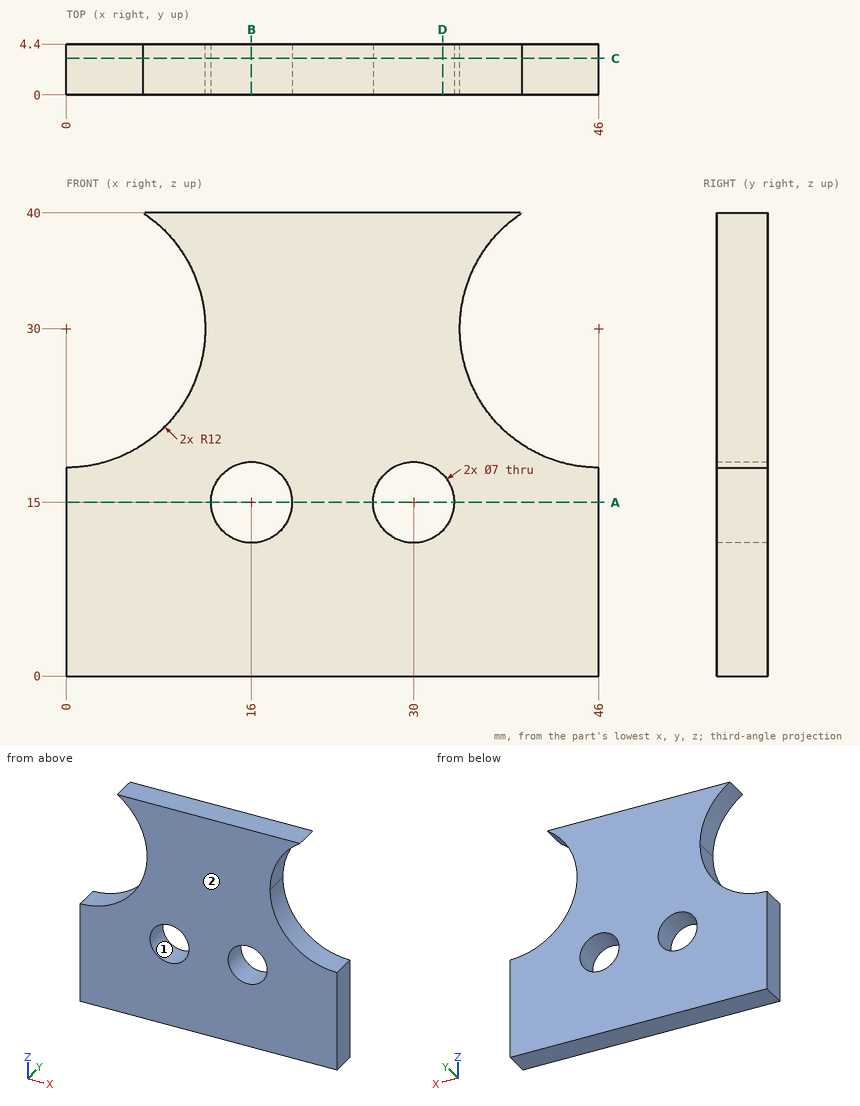
Print and shaded views of the part. All mm, measured from the part's lowest x, y and z. Round coordinates to 2 decimals unless told otherwise and drop trailing zeros. Write each loop counter-clockwise with the first axis right and the second up, starting at its lowest first coordinate (ties: lowest second). Pieces come first, ordered by that corner, then holes.
Item 1: Two-plate mould, pull along X, no slides. Class the marked faces 1 and 2: +X half, -X half, draft (parallel to the pull), parting line (faces both ways), or undercut.
Results:
face 1: undercut
face 2: draft
Item 2: Cut at B-B, the plane x = 16. Give the cut face in (y, z).
Results:
outline: (0, 0) - (4.4, 0) - (4.4, 11.5) - (0, 11.5) - close; (0, 18.5) - (4.4, 18.5) - (4.4, 40) - (0, 40) - close
Item 3: Probe L1, parallel to X at y = 3.5, z = 15; L2, parallel to Z at x = 37, y = 1.55; L3, parallel to Z at x = 8.5, y = 1.2. List the from-to ranges inside material, lowest first.
Results:
L1: x = 0 to 12.5, 19.5 to 26.5, 33.5 to 46
L2: z = 0 to 22.06, 37.94 to 40
L3: z = 0 to 21.53, 38.47 to 40
Item 4: Cut at A-A, the plane z = 15. Give the cut face in (x, y), plus the area to 3 significant figures.
Results:
outline: (0, 0) - (12.5, 0) - (12.5, 4.4) - (0, 4.4) - close; (19.5, 0) - (26.5, 0) - (26.5, 4.4) - (19.5, 4.4) - close; (33.5, 0) - (46, 0) - (46, 4.4) - (33.5, 4.4) - close
area: 141 mm2
Item 5: Cut at D-D, the plane x = 32.5. Give the cut face in (y, z), plus the area to 3 significant figures.
Results:
outline: (0, 0) - (4.4, 0) - (4.4, 12.55) - (0, 12.55) - close; (0, 17.45) - (4.4, 17.45) - (4.4, 40) - (0, 40) - close
area: 154 mm2
Item 6: Cut at C-C, the plane y = 3.15. Give the cut face in (x, z), plus the area to 3 significant figures.
Results:
outline: (0, 0) - (46, 0) - (46, 18) arc R12 cw to (39.37, 40) - (6.63, 40) arc R12 cw to (0, 18) - close; hole circle Ø7 at (16, 15); hole circle Ø7 at (30, 15)
area: 1,330 mm2
